```python
from build123d import *

# Parameters (mm, degrees)
SKETCH1_W               = 29
SKETCH1_H               = 10
BOSS_EXTRUDE1_DEPTH     = 5
SKETCH2_R               = 2.413
CUT_EXTRUDE1_DEPTH      = 17.132265805
SKETCH3_R               = 1.27
CUT_EXTRUDE2_DEPTH      = 17.132265805
SKETCH4_R               = 1.8669
CUT_EXTRUDE3_DEPTH      = 1.524
CUT_EXTRUDE4_REACH      = 19.524
CUT_EXTRUDE4_END_RADIUS = 1.27
SKETCH5_R               = 1.143


with BuildPart() as part:
    # Sketch1 → Boss-Extrude1 (new body)
    with BuildSketch(Plane.XY):
        Rectangle(SKETCH1_W, SKETCH1_H)
    extrude(amount=BOSS_EXTRUDE1_DEPTH)

    # Sketch2 → Cut-Extrude1 (cut, through all)
    with BuildSketch(Plane.XY.offset(5)):
        with Locations((-9.5, 0)):
            Circle(SKETCH2_R)
        with Locations((9.5, 0)):
            Circle(SKETCH2_R)
    extrude(amount=-CUT_EXTRUDE1_DEPTH, mode=Mode.SUBTRACT)

    # Sketch3 → Cut-Extrude2 (cut, through all)
    with BuildSketch(Plane.XY.offset(5)):
        Circle(SKETCH3_R)
    extrude(amount=-CUT_EXTRUDE2_DEPTH, mode=Mode.SUBTRACT)

    # Sketch4 → Cut-Extrude3 (cut)
    with BuildSketch(Plane(origin=(0, 5, 0), x_dir=(1, 0, 0), z_dir=(0, 1, 0))):
        with Locations(Location((0, -2.5, 0), (0, 0, 180))):
            Circle(SKETCH4_R)
    extrude(amount=-CUT_EXTRUDE3_DEPTH, mode=Mode.SUBTRACT)

    # Cut-Extrude4: up to this cylinder (the profile starts outside it)
    cut_extrude4_end = Plane(origin=(0, 0, 2.5), z_dir=(0, 0, 1)) * Cylinder(CUT_EXTRUDE4_END_RADIUS, 42.588, mode=Mode.PRIVATE)
    # Sketch5 → Cut-Extrude4 (cut, up to the surface)
    with BuildSketch(Plane(origin=(0, 3.476, 0), x_dir=(1, 0, 0), z_dir=(0, 1, 0)), mode=Mode.PRIVATE) as cut_extrude4_sk1:
        with Locations(Location((0, -2.5, 0), (0, 0, 180))):
            Circle(SKETCH5_R)
    cut_extrude4_tool1 = extrude(cut_extrude4_sk1.sketch, amount=-CUT_EXTRUDE4_REACH, mode=Mode.PRIVATE) - cut_extrude4_end
    add(cut_extrude4_tool1.solids().sort_by_distance((0, 3.476, 2.5))[0], mode=Mode.SUBTRACT)


solid = part.part
```
The model under review builds one solid part; all positions refer to its coordinate system, in mm. A direction names the side the tool comes from. Give positions to 0.01 mm unless a question says otherwise; leave off trailing zeros. Write each loop counter-clockwise with the first axis right and the second up, starting at its lowest first coordinate (ties: lowest second). Pieces come first, ordered by that corner, then holes. Notation, with made-up numbers: M -7,72 L 19,72 A14 ccw 19,95 Z; hole C 63.5,36.25 d3. An arc over 180 degrees is marked long. Answer in a Markdown table with one row per item.
Item 1: Draft analysis for pull direction Z (two halves, no side actions). For faces 1 (the face through (0, -5, 2)), 2 (the face through (0, 2, 5)), 3 (the face through (-1.09, 2.36, 2.84)), state which applies: +Z half, -Z half, draft (parallel to the pull), parting line (faces both ways), or undercut.
Check sheet entries:
| item | result |
|---|---|
| face 1 | draft |
| face 2 | +Z half |
| face 3 | undercut |
Item 2: Add section C-C on z = 2.5. Give the boundary of the cut face in (x, y).
Check sheet entries:
| item | result |
|---|---|
| outline | M -14.5,-5 L 14.5,-5 L 14.5,5 L 1.87,5 L 1.87,3.48 L 1.14,3.48 L 1.14,0.55 A1.27 cw long -1.14,0.55 L -1.14,3.48 L -1.87,3.48 L -1.87,5 L -14.5,5 Z; hole C -9.5,0 d4.83; hole C 9.5,0 d4.83 |
Item 3: Add section D-D on y = 1.75. Give the boundary of the cut face in (x, z).
Check sheet entries:
| item | result |
|---|---|
| outline | M -14.5,0 L -11.16,0 L -11.16,5 L -14.5,5 Z; M -7.84,0 L 7.84,0 L 7.84,5 L -7.84,5 Z; M 11.16,0 L 14.5,0 L 14.5,5 L 11.16,5 Z; hole C 0,2.5 d2.29 |
Item 4: Tool access review of faces 4 (the face through (14.5, 0, 2)), 5 (the face through (0, 3.476, 1)): name each direction out of +Z, -Z, +X, -X, +Y, -Y from which nothing blocks a thin tool from reaching the whole face with its end or side.
Check sheet entries:
| item | result |
|---|---|
| face 4 | +Z, -Z, +X, +Y, -Y |
| face 5 | +Y |
Item 5: For line 1 along Y through (x, z) = (9.5, 3.6); line 2 along Z through (x, y) = (0, 1.6); line 3 along X through (y, z) = (1.55, 2.5), list the stretches that pass through material, from the lowest coordinate up.
Check sheet entries:
| item | result |
|---|---|
| line 1 | -5 to -2.41, 2.41 to 5 |
| line 2 | 0 to 1.36, 3.64 to 5 |
| line 3 | -14.5 to -11.35, -7.65 to -1.14, 1.14 to 7.65, 11.35 to 14.5 |
Item 6: Add section B-B on y = 0. Give the boundary of the cut face in (x, z), plus the area to 3 significant figures.
Check sheet entries:
| item | result |
|---|---|
| outline | M -14.5,0 L -11.91,0 L -11.91,5 L -14.5,5 Z; M -7.09,0 L -1.27,0 L -1.27,5 L -7.09,5 Z; M 1.27,0 L 7.09,0 L 7.09,5 L 1.27,5 Z; M 11.91,0 L 14.5,0 L 14.5,5 L 11.91,5 Z |
| area | 84.0 mm2 |
Item 7: For P1, Ø2, axis at x = 0, z = 2.5, coming from the +Y side, flat-tipped, find the tip position at first contact; note if it passes through.
Check sheet entries:
| item | result |
|---|---|
| P1 | y = -0.78 |
Item 8: Add section A-A on x = 9.5. Give the boundary of the cut face in (y, z), plus the area to 3 significant figures.
Check sheet entries:
| item | result |
|---|---|
| outline | M -5,0 L -2.41,0 L -2.41,5 L -5,5 Z; M 2.41,0 L 5,0 L 5,5 L 2.41,5 Z |
| area | 25.9 mm2 |
